Verification items for the finished model (mm, model axes). Face numbers are marked on the shaded views. A direction names the side the tool comes from. Give positions to 0.01 mm unless a question says otherwise; leave off trailing zeros. Order: outer loops, then holes, each group sorted by start corner. A loop starts at its lowest first (then second) coordinate and runs counter-clockwise, first axis right, second up. Notation, with made-up numbers: (38.25, 64.25) - (58.25, 64.25) arc R20 ccw to (58.25, 68.25) - close; hole circle Ø6 at (85, 18.5). An arc over 180 degrees is marked (long way). Answer as a JSON object with one key per item and string values. Group by question number.
(1) Section check B-B (z = 0). Record the boundary of the cut face in (x, y), then the cut area to 3 significant figures.
(2) Depth check by flat-ended pin: pin 1 Ø2 at (x, z) = (-4, 1.5) entering from +Y; pin 2 Ø1.5 at (x, z) = (-5, -1) entering from -Y; pin 3 Ø1.5 at (y, z) = (-5, 2.5) entering from -X. Enter the tip coordinate at first touch or a pass-through.
(3) Access from +Z, -Z, +X, -X, +Y, -Y to the whole of each face (thin tool, end or side, straight path). Record for the marked faces 1 and 2.
(4) Section check A-A (y = 0). Record the boundary of the cut face in (x, z), then the cut area to 3 significant figures.
(5) Thickness scan on line 1 (X direction, y = -5.25, z = -2.5); line 2 (X direction, y = -6, z = -2.5); line 3 (Z direction, x = 8, y = 4). Record the ranges inside material, lowest first.
Autodesk Inventor part; units mm, degrees
ref_plane "YZ Plane" through (0, 0, 0) normal (1, 0, 0) x (0, 1, 0)
ref_plane "XZ Plane" through (0, 0, 0) normal (0, 1, 0) x (-1, 0, 0)
ref_plane "XY Plane" through (0, 0, 0) normal (0, 0, 1) x (1, 0, 0)
sketch "Sketch1" plane through (0, 0, 0) normal (0, 0, 1) x (1, 0, 0)
  circle A0 centre (0, 0) radius 8
  dimension "d0" = 16
extrude "Extrusion1" add sketch "Sketch1" along normal mid plane 6
fillet "Fillet1" radius 1 2 edges at (-8, 0, 3) (-8, 0, -3)
sketch "Sketch2" plane through (0, 0, 0) normal (1, 0, 0) x (0, 1, 0)
  circle A0 centre (3.9, 1.9) radius 0.75
  circle A1 centre (-3.9, -1.9) radius 0.75
  point P0 (0, 0)
  dimension "d4" = 3.9
  dimension "d5" = 3.9
  dimension "d8" = 1.5
  dimension "d9" = 1.5
  dimension "d20" = 1.9
  dimension "d21" = 1.9
extrude "Extrusion2" add sketch "Sketch2" along normal blind 10
sketch "Sketch3" plane through (10, 3.9, 1.9) normal (1, 0, 0) x (0, 0, -1)
  circle A0 centre (0, 0) radius 0.4
  circle A1 centre (3.8, -7.8) radius 0.4
  point P0 (1.9, -3.9)
  dimension "d14" = 3.9
  dimension "d15" = 3.9
  dimension "d16" = 0.8
  dimension "d17" = 0.8
  dimension "d22" = 1.9
  dimension "d23" = 1.9
extrude "Extrusion3" add sketch "Sketch3" along normal blind 4
properties part number "16mm_7_2mmDiskPTC"
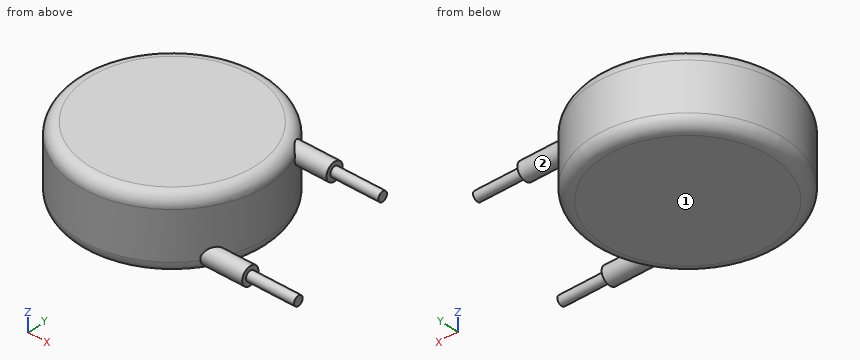
Solutions:
{
 "1": {"outline": "circle Ø16 at (0, 0)", "area": "201 mm2"},
 "2": {"pin 1": "stops at y = 7.42", "pin 2": "stops at y = -6.78", "pin 3": "stops at x = -6.71"},
 "3": {"face 1": "-Z, +X, -X, +Y, -Y", "face 2": "+X"},
 "4": {"outline": "(-8, -2) arc R1 ccw to (-7, -3) - (7, -3) arc R1 ccw to (8, -2) - (8, 2) arc R1 ccw to (7, 3) - (-7, 3) arc R1 ccw to (-8, 2) - close", "area": "95.1 mm2"},
 "5": {"line 1": "x = -5.86 to 5.86", "line 2": "x = -5.09 to 5.09", "line 3": "z = 1.16 to 2.64"}
}
